from build123d import *

# Parameters (mm, degrees)
F0_W     = 0.635
F0_H     = 5.461
F2_DEPTH = 3.175


with BuildPart() as f1:
    # F0 (on Front) → F1 (revolve)
    with BuildSketch(Plane.XZ):
        with BuildLine():
            Line((0, 0), (7.62, 0))
            Line((7.62, 0), (7.62, 1.651))
            Line((7.62, 1.651), (6.35, 1.651))
            Line((6.35, 1.651), (6.35, 5.842))
            Line((6.35, 5.842), (6.290507, 5.842))
            ThreePointArc((6.290507, 5.842), (6.276233, 5.846566), (6.267258, 5.858569))
            Line((6.267258, 5.858569), (4.826, 10.033))
            Line((4.826, 10.033), (4.826, 10.922))
            Line((4.826, 10.922), (5.207, 10.922))
            Line((5.207, 10.922), (5.207, 12.573))
            Line((5.207, 12.573), (3.175, 12.573))
            Line((3.175, 12.573), (3.175, 14.224))
            Line((3.175, 14.224), (2.413, 14.224))
            Line((2.413, 14.224), (2.413, 19.685))
            Line((2.413, 19.685), (0.635, 19.685))
            Line((0.635, 19.685), (0.635, 14.224))
            Line((0.635, 14.224), (0, 14.224))
            Line((0, 14.224), (0, 0))
        make_face()
    revolve(axis=Axis((0, 0, 13.806538), (0, 0, -1)))

    # F0 (on Front) → F2 (cut, symmetric)
    with BuildSketch(Plane.XZ):
        with Locations((-0.3175, 16.9545)):
            Rectangle(F0_W, F0_H)
        with Locations((0.3175, 16.9545)):
            Rectangle(F0_W, F0_H)
    extrude(amount=F2_DEPTH, both=True, mode=Mode.SUBTRACT)


solid = f1.part
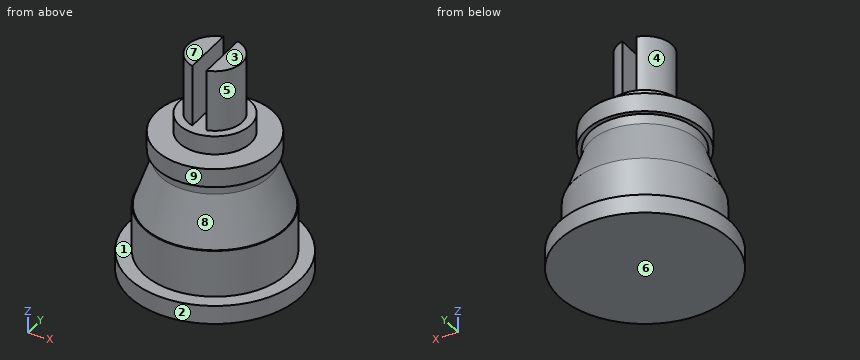
Model file for the job. Use its own axes, mm. Face numbers are marked on the shaded views. A direction names the side the tool comes from. Round coordinates to 2 decimals unless told otherwise and drop trailing zeros. Loops run counter-clockwise (first coordinate to the right, second up) from the corner with the lowest first, then second, coordinate; pieces in that order, holes last. Notation, with made-up numbers: (39.25, 70) - (48.25, 70) arc R34 cw to (48.25, 107) - close; hole circle Ø5 at (82.25, -36). An arc over 180 degrees is marked (long way). Write each question's results on one line, items separated by ' | '.
(1) Pin check, flat tips, straight feed: pin 1 (3.5 mm diameter, centred on y = -1, z = 18, fed in from +X); pin 2 (4 mm diameter, centred on y = -3.5, z = 11.5, fed in from -X); pin 3 (4 mm diameter, centred on y = -5.5, z = 12.5, fed in from -X). Stop position of each tip, or through.
Answer below:
pin 1: stops at x = 2.41 | pin 2: stops at x = -4.99 | pin 3: stops at x = -3.86
(2) Saw through at C-C, the plane z = 16. List the corners of the cut face in (x, y) (3 decimals), then the cut area to 3 significant figures.
Answer below:
outline: (-0.635, -2.328) - (-0.635, 2.328) arc R2.413 ccw to start; (0.635, -2.328) arc R2.413 ccw to (0.635, 2.328) - close | area: 12.2 mm^2
(3) Wall check: L1, parallel to Z at x = -3.25, y = -1.5; L2, parallel to Z at x = 3.5, y = -5.75; L3, parallel to X at y = 0.25, z = 14.75 (3 decimals). Give the ranges that are in metal, low to high.
Answer below:
L1: z = 0 to 12.57 | L2: z = 0 to 1.65 | L3: x = -2.4 to -0.635, 0.635 to 2.4
(4) Mould opens along Z. For the marked faces 6, 7, 8 and 9 say: released by +Z, released by -Z, zero draft, split by the parting line, or undercut.
Answer below:
face 6: released by -Z | face 7: released by +Z | face 8: undercut | face 9: zero draft
(5) Saw through at D-D, the plane z = 6.25. List the corners of the cut face in (x, y).
Answer below:
outline: circle Ø12.26 at (0, 0)
(6) 3-axis set-ups, long thin cutter, end or side, ignore diameter. For the marked faces 1, 2, 3, 4 and 5: which of +Z, -Z, +X, -X, +Y, -Y reach the whole face in a straight line?
Answer below:
face 1: +Z | face 2: +Z, -Z | face 3: +Z, +X, -X, +Y, -Y | face 4: +Z, -X | face 5: +Z, +X
